Input: part model. Units: mm. Frame: model coordinates. A direction names the side the tool comes from. Give positions to 0.01 mm unless a question says otherwise; leave off trailing zeros. Loops run counter-clockwise (first coordinate to the right, second up) from the corner with the lowest first, then second, coordinate; pieces in that order, holes last. Notation, with made-up numbers: (47, -36.5) -> (55, -36.5) arc R25 ccw to (55, -12.5) -> close; hole circle Ø10 at (64, -38). An arc over 180 degrees is marked (long way). One line per question, with ' | ' between items.
from build123d import *

# Parameters (mm, degrees)
SKETCH1_W              = 19
SKETCH1_H              = 9
SKETCH1_R              = 1.8
BOSS_EXTRUDE1_DEPTH    = 4.8
BOSS_EXTRUDE1_2_DEPTH  = 4.8
BOSS_EXTRUDE1_3_DEPTH  = 4.8
SKETCH1_W_2            = 18.947549714
BOSS_EXTRUDE1_4_DEPTH  = 4.8
BOSS_EXTRUDE2_DEPTH    = 4
BOSS_EXTRUDE3_DEPTH    = 8
BOSS_EXTRUDE4_DEPTH    = 8
FILLET1_R              = 2.8
SKETCH11_W             = 19
SKETCH11_H             = 4.8
BOSS_EXTRUDE5_DEPTH    = 3
BOSS_EXTRUDE6_DEPTH    = 3
LPATTERN1_COUNT        = 2
LPATTERN1_PITCH        = 157
CUT_EXTRUDE2_START     = -4
CUT_EXTRUDE2_OUTLINE_W = 6.933333333
CUT_EXTRUDE2_OUTLINE_H = 40
CUT_EXTRUDE2_DEPTH     = 4
SKETCH12_W             = 19
SKETCH12_H             = 4.8
BOSS_EXTRUDE7_DEPTH    = 3
SKETCH12_4_W           = 8
SKETCH12_4_H           = 18.8
BOSS_EXTRUDE9_DEPTH    = 3


# Read off the part's stored shape, not the designer's step: Cut-Extrude2
with BuildPart() as part:
    # Sketch1 → Boss-Extrude1 (new body)
    with BuildSketch(Plane.XY):
        with Locations((80, 58.45)):
            Rectangle(SKETCH1_W, SKETCH1_H)
        with Locations(Location((78.5, 57.45, 0), (0, 0, 180))):
            Circle(SKETCH1_R, mode=Mode.SUBTRACT)
    extrude(amount=-BOSS_EXTRUDE1_DEPTH)



with BuildPart() as body_2:
    # Sketch1 → Boss-Extrude1 2 (new body)
    with BuildSketch(Plane.XY):
        with Locations((80, -58.45)):
            Rectangle(SKETCH1_W, SKETCH1_H)
        with Locations((78.5, -57.45)):
            Circle(SKETCH1_R, mode=Mode.SUBTRACT)
    extrude(amount=-BOSS_EXTRUDE1_2_DEPTH)

    # Sketch12 → Boss-Extrude7 (add)
    with BuildSketch(Plane.XZ.offset(62.95)):
        Polygon((70.5, -4.8), (70.5, 0), (62.5, 0), (62.5, -18.8), (70.5, -18.8), align=None)
        Polygon((70.5, -18.8), (89.5, -4.8), (70.5, -4.8), align=None)
        with Locations((80, -2.4)):
            Rectangle(SKETCH12_W, SKETCH12_H)
        Polygon((-86.5, -18.8), (-67.552450286, -4.8), (-67.552450286, 0), (-94.5, 0), (-94.5, -18.8), align=None)
    extrude(amount=BOSS_EXTRUDE7_DEPTH)


with BuildPart() as body_3:
    # Sketch1 → Boss-Extrude1 3 (new body)
    with BuildSketch(Plane.XY):
        with Locations((-77, 58.45)):
            Rectangle(SKETCH1_W, SKETCH1_H)
        with Locations((-78.5, 57.45)):
            Circle(SKETCH1_R, mode=Mode.SUBTRACT)
    extrude(amount=-BOSS_EXTRUDE1_3_DEPTH)


with BuildPart() as body_4:
    # Sketch1 → Boss-Extrude1 4 (new body)
    with BuildSketch(Plane.XY):
        with Locations((-77.026225143, -58.448744181)):
            Rectangle(SKETCH1_W_2, SKETCH1_H)
        with Locations(Location((-78.5, -58.45, 0), (0, 0, 180))):
            Circle(SKETCH1_R, mode=Mode.SUBTRACT)
    extrude(amount=-BOSS_EXTRUDE1_4_DEPTH)


with BuildPart() as body_5:
    # Sketch3 → Boss-Extrude2 (new body)
    with BuildSketch(Plane(origin=(0, 0, -14.8), x_dir=(-1, 0, 0), z_dir=(0, 0, -1))):
        with BuildLine():
            Line((-77.5, -50), (82.5, -50))
            Line((82.5, -50), (86.5, -50))
            Line((86.5, -50), (86.5, 50))
            Line((86.5, 50), (82.5, 50))
            Line((82.5, 50), (-77.5, 50))
            ThreePointArc((-77.5, 50), (-81.035533906, 48.535533906), (-82.5, 45))
            Line((-82.5, 45), (-82.5, -45))
            ThreePointArc((-82.5, -45), (-81.035533906, -48.535533906), (-77.5, -50))
        make_face()
    extrude(amount=BOSS_EXTRUDE2_DEPTH)


with BuildPart() as part_1:
    add(part.part)

    add(body_5.part)  # Boss-Extrude3 merges body 5
    # Sketch4 → Boss-Extrude3 (add)
    with BuildSketch(Plane.ZY.offset(-70.5)):
        Polygon((-18.8, 61.95), (-18.8, 50), (-14.8, 50), (-14.8, 53.95), (0, 53.95), (0, 61.95), align=None)
    boss_extrude3 = extrude(amount=BOSS_EXTRUDE3_DEPTH)

    # Mirror4: Boss-Extrude3 across plane
    add(boss_extrude3.mirror(Plane.ZX))


    add(body_3.part)  # Boss-Extrude4 merges body 3

    add(body_4.part)  # Boss-Extrude4 merges body 4
    # Sketch10 → Boss-Extrude4 (add)
    with BuildSketch(Plane.ZY.offset(86.5)):
        Polygon((-14.8, 50), (-14.8, 26.95), (-14.8, -50), (-14.8, -53.95), (0, -53.95), (0, -61.95), (-18.8, -61.95), (-18.8, -50), (-18.8, 26.95), (-18.8, 50), (-18.8, 61.95), (0, 61.95), (0, 53.95), (-14.8, 53.95), align=None)
    extrude(amount=BOSS_EXTRUDE4_DEPTH)

    # Fillet1
    fillet1_edges = [part_1.edges().sort_by_distance(p)[0] for p in [
        (62.5, 50, -16.8),
        (70.5, 50, -16.8),
        (-86.5, 50, -16.8),
        (62.5, -50, -16.8),
        (-86.5, -50, -16.8),
        (70.5, -50, -16.8),
    ]]
    fillet(fillet1_edges, radius=FILLET1_R)

    # Sketch11 → Boss-Extrude5 (add)
    with BuildSketch(Plane(origin=(0, 62.95, 0), x_dir=(1, 0, 0), z_dir=(0, 1, 0))):
        with Locations((80, 2.4)):
            Rectangle(SKETCH11_W, SKETCH11_H)
        Polygon((89.5, 4.8), (70.5, 18.8), (70.5, 4.8), align=None)
    boss_extrude5 = extrude(amount=BOSS_EXTRUDE5_DEPTH)

    # Sketch11<5> → Boss-Extrude6 (add, symmetric)
    with BuildSketch(Plane(origin=(0, 62.95, 0), x_dir=(1, 0, 0), z_dir=(0, 1, 0))):
        Polygon((62.5, 18.8), (62.5, 0), (70.5, 0), (70.5, 4.8), (70.5, 18.8), align=None)
    boss_extrude6 = extrude(amount=BOSS_EXTRUDE6_DEPTH, both=True)

    # LPattern1: Boss-Extrude5, Boss-Extrude6 ×2
    with Locations(*[(-i * LPATTERN1_PITCH, 0, 0) for i in range(1, LPATTERN1_COUNT)]):
        add(boss_extrude5)
        add(boss_extrude6)

    # Cut-Extrude2 outline → Cut-Extrude2 (cut)
    with BuildSketch(Plane(origin=(0, 0, -18.8), x_dir=(-1, 0, 0), z_dir=(0, 0, -1)).offset(CUT_EXTRUDE2_START)):
        with BuildLine():
            add(Edge.make_bspline(
                [(10.975, -14.666666667), (10.853422825, -14.380277897), (10.602565639, -13.789355455), (10.2019734, -12.881204225), (9.767405766, -11.924663917), (9.307519179, -10.914258143), (8.824913039, -9.84726331), (8.314703241, -8.72434694), (7.79171958, -7.538855775), (7.060810636, -5.888109041), (6.129555226, -3.804410061), (4.927921427, -1.367968701), (3.745344455, 1.001863959), (2.800332488, 2.930787983), (2.085444913, 4.420434389), (1.562508134, 5.460457627), (1.061997748, 6.444961947), (0.646894723, 7.213714992), (0.390028809, 7.741258394), (0.294400491, 7.960576425), (0.265045842, 8.033579646)],
                knots=[0, 0, 0, 0, 0.034500563, 0.071187, 0.110063316, 0.15100446, 0.194290954, 0.239922853, 0.287774458, 0.337971758, 0.440120704, 0.540825287, 0.639182399, 0.733823363, 0.779010204, 0.822402877, 0.862904814, 0.901482229, 0.919254697, 0.927976768, 0.927976768, 0.927976768, 0.927976768], degree=3))
            Line((10.975, -14.666666667), (16.433333333, -14.666666667))
            add(Edge.make_bspline(
                [(27.185837823, 8.182370431), (27.16617885, 8.135201447), (27.077190149, 7.929706006), (26.638721231, 7.048600418), (25.829878755, 5.497567499), (24.783516915, 3.316615567), (23.677292972, 1.061322281), (22.496472017, -1.232864568), (21.307452474, -3.637070323), (20.375347087, -5.74013551), (19.642877201, -7.45328115), (19.114948929, -8.684692719), (18.595469257, -9.83506941), (18.101022183, -10.910308731), (17.641251792, -11.924811954), (17.206280513, -12.881167962), (16.805785724, -13.789363687), (16.554916393, -14.380280585), (16.433333333, -14.666666667)],
                knots=[0.069075624, 0.069075624, 0.069075624, 0.069075624, 0.074722211, 0.093815852, 0.177875914, 0.268118698, 0.361243693, 0.455604817, 0.553401566, 0.65774291, 0.709886229, 0.759408515, 0.805872658, 0.849438848, 0.8902598, 0.929021986, 0.965600721, 1, 1, 1, 1], degree=3))
            add(Edge.make_bspline(
                [(28.416666667, -20), (28.370326707, -18.622190652), (28.278576595, -15.894217539), (28.126835921, -11.841493191), (27.972919305, -7.871719916), (27.793529228, -4.002689262), (27.621652056, -0.271985015), (27.446461619, 3.283575307), (27.301676648, 6.080429142), (27.213112404, 7.691042727), (27.185837823, 8.182370431)],
                knots=[0, 0, 0, 0, 0.138334797, 0.273893922, 0.406956967, 0.536980294, 0.66254851, 0.781713115, 0.894196585, 0.943574943, 0.943574943, 0.943574943, 0.943574943], degree=3))
            Line((28.416666667, -20), (35.333333333, -20))
            add(Edge.make_bspline(
                [(32.608333333, 20), (32.900086832, 16.750700945), (33.488285429, 10.199851855), (34.22240543, 0.281966095), (34.854498798, -9.801801427), (35.172888466, -16.58285171), (35.333333333, -20)],
                knots=[0, 0, 0, 0, 0.244084907, 0.492094869, 0.744053343, 1, 1, 1, 1], degree=3))
            Line((32.608333333, 20), (26.5, 20))
            add(Edge.make_bspline(
                [(13.708333333, -7.2), (13.830007974, -6.723206803), (14.084227403, -5.727024743), (14.60790834, -4.202590997), (15.228118515, -2.563650948), (16.267159704, -0.227490136), (17.691281094, 2.819546572), (19.414993101, 6.558422585), (21.178315261, 10.255040247), (22.694244718, 13.223986219), (23.88002457, 15.483108195), (24.769643789, 17.058555357), (25.620362017, 18.56810669), (26.210964283, 19.529501548), (26.5, 20)],
                knots=[0, 0, 0, 0, 0.048991334, 0.102359448, 0.160419925, 0.223485875, 0.356930682, 0.495438602, 0.633536698, 0.764814667, 0.827438497, 0.887631747, 0.945007934, 1, 1, 1, 1], degree=3))
            add(Edge.make_bspline(
                [(0.875, 20), (1.488654305, 18.979646564), (2.747485512, 16.886525506), (4.528875905, 13.57233268), (6.317629783, 10.03594448), (8.05073889, 6.322134495), (9.762822193, 2.612044415), (11.165454408, -0.380308514), (12.190165242, -2.648246106), (12.811441851, -4.240209855), (13.334558303, -5.740131954), (13.586944811, -6.725888004), (13.708333333, -7.2)],
                knots=[0, 0, 0, 0, 0.118514609, 0.243117155, 0.374451296, 0.51299163, 0.651063123, 0.781216145, 0.842002695, 0.898745008, 0.951300115, 1, 1, 1, 1], degree=3))
            Line((0.875, 20), (-5.15, 20))
            add(Edge.make_bspline(
                [(-7.866666667, -20), (-7.793061043, -18.169390935), (-7.648961945, -14.585573542), (-7.412691767, -9.29864876), (-7.122844657, -4.171204641), (-6.81303939, 0.843509011), (-6.445549688, 5.747929795), (-6.081795853, 10.555682601), (-5.642721893, 15.291472548), (-5.314200688, 18.430872547), (-5.15, 20)],
                knots=[0, 0, 0, 0, 0.137063101, 0.268330979, 0.395915623, 0.521267524, 0.644201892, 0.763852071, 0.881969103, 1, 1, 1, 1], degree=3))
            Line((-7.866666667, -20), (-0.966666667, -20))
            add(Edge.make_bspline(
                [(0.265045842, 8.033579646), (0.240657124, 7.594605286), (0.154028006, 6.039024937), (-0.000810917, 3.297839119), (-0.167059263, -0.255673004), (-0.358502841, -3.988239018), (-0.518551576, -7.860926765), (-0.678215675, -11.835877361), (-0.828073098, -15.891460777), (-0.92018915, -18.622196537), (-0.966666667, -20)],
                knots=[0.061407132, 0.061407132, 0.061407132, 0.061407132, 0.105523386, 0.217741555, 0.336904218, 0.462483689, 0.592771123, 0.725832, 0.861667458, 1, 1, 1, 1], degree=3))
        make_face()
        with Locations((45.733333333, 0)):
            Rectangle(CUT_EXTRUDE2_OUTLINE_W, CUT_EXTRUDE2_OUTLINE_H)
        Polygon((-29.2, 20), (-36.133333333, 20), (-36.133333333, -20), (-11.066666667, -20), (-11.066666667, -14.666666667), (-29.2, -14.666666667), align=None)
    extrude(amount=CUT_EXTRUDE2_DEPTH, mode=Mode.SUBTRACT)



with BuildPart() as boss_extrude7_piece_1:
    # of the separate pieces the step leaves, piece 1, a body of its own (boss_extrude7_pieces)
    add(body_2.part.solids().sort_by_distance((89.5, -53.95, 0))[0])


with BuildPart() as boss_extrude7_piece_2:
    # of the separate pieces the step leaves, piece 2, a body of its own (boss_extrude7_pieces)
    add(body_2.part.solids().sort_by_distance((-86.5, -62.95, -18.8))[0])


with BuildPart() as part_2:
    add(part_1.part)

    add(boss_extrude7_piece_1.part)  # Boss-Extrude9 merges Boss-Extrude7 piece 1

    add(boss_extrude7_piece_2.part)  # Boss-Extrude9 merges Boss-Extrude7 piece 2
    # Sketch12<4> → Boss-Extrude9 (add)
    with BuildSketch(Plane.XZ.offset(62.95)):
        with Locations((-90.5, -9.4)):
            Rectangle(SKETCH12_4_W, SKETCH12_4_H)
        Polygon((70.5, -4.8), (70.5, 0), (62.5, 0), (62.5, -18.8), (70.5, -18.8), align=None)
    extrude(amount=-BOSS_EXTRUDE9_DEPTH)


solid = part_2.part
1. Section query B-B (z = -2.25). Count the separate pieces of the cut face and the enclosed holes in it, then the cut area to 3 significant figures.
Determined:
separate pieces: 4 | enclosed holes: 4 | area: 1,250 mm2
2. Pull-direction query (X, two-part tool) for faces 6 (the cylindrical face through (-78.11, -56.693, -2.366)), 7 (the flat face through (-77, -53.949, -2)), 8 (the flat face through (89.5, 60, -2)), 9 (the flat face through (-77, -60, -4.8)); classes: pulls with the +X half, pulls with the -X half, needs draft (parallel to the pull), parting line crosses it, or undercut.
Determined:
face 6: undercut | face 7: needs draft | face 8: pulls with the +X half | face 9: undercut
3. Pin query (flat end, axial travel): P1, Ø3, axis at y = 5.5, z = -17.5, coming from the +X side; P2, Ø1.2, axis at x = 3.5, z = -16.5, coming from the +Y side; P3, Ø2, axis at y = -15, z = -12.5, coming from the -X side. Return the tip coordinate at first contact, or that it passes through.
Determined:
P1: stops at x = 82.5 | P2: stops at y = 50 | P3: passes through
4. Section query A-A (x = 27). Output: boundary loops of the cut face in (y, z), then the cut area to 3 significant figures.
Determined:
outline: (-50, -18.8) -> (-20, -18.8) -> (-20, -14.8) -> (-50, -14.8) -> close; (-14.67, -18.8) -> (50, -18.8) -> (50, -14.8) -> (-14.67, -14.8) -> close | area: 379 mm2
5. Section query C-C (x = 57.5). Output: boundary loops of the cut face in (y, z).
Determined:
outline: (-50, -18.8) -> (50, -18.8) -> (50, -14.8) -> (-50, -14.8) -> close
6. Ray query, line 1 along Y through (x, z) = (78.5, -1); line 2 along X through (y, z) = (61.5, -18); line 3 along Z through (x, y) = (-80, -31.5). Return the intervals inside material, ascending. Write a range as from..to.
Determined:
line 1: y = -65.95..-59.25, -55.65..-53.95, 53.95..55.65, 59.25..65.95 | line 2: x = -94.5..-86.5, 62.5..70.5 | line 3: z = -18.8..-14.8
7. Reachability of faces 1 (the flat face through (80.133, 64.429, -11.702)), 2 (the flat face through (75, 50, -17)), 3 (the flat face through (-86.5, -58, -12)), 4 (the flat face through (70.5, 58, -12)), 5 (the flat face through (-5, -13, -14.8)) from +Z, -Z, +X, -X, +Y, -Y: full face, straight path, thin tool, end or side. Return the list, or none.
Determined:
face 1: -Z, +X, +Y | face 2: +Z, -Z, +X | face 3: -Z | face 4: -Z, +X | face 5: +Z, +X, -X
